CAD build for the part. Positions are in the model's coordinates, mm. A direction names the side the tool comes from. Give positions to 0.01 mm unless a question says otherwise; leave off trailing zeros. Loops run counter-clockwise (first coordinate to the right, second up) from the corner with the lowest first, then second, coordinate; pieces in that order, holes last. Notation, with made-up numbers: M -15.5,82 L -7.5,82 A20 cw -7.5,104 Z; hole C 26.25,-35 d3. An arc over 180 degrees is marked long. One line per question, with ' | ' between items.
```python
from build123d import *

# Parameters (mm, degrees)
F0_R     = 5
F1_DEPTH = 4
F2_DEPTH = 2
F0_R_2   = 2
F3_DEPTH = 16
F4_SIZE  = 0.75
F5_SIZE  = 0.75


with BuildPart() as f1:
    # F0 (on Top) → F1 (new body)
    with BuildSketch(Plane.XY):
        Polygon((-4.5, 20.5), (-4.5, 17.5), (-1.8038475773, 17.5), (-3.375, 18.4071052742), (-3.375, 20.5), align=None)
        Polygon((3.875, 18.4071052742), (2.3038475773, 17.5), (5, 17.5), (5, 20.5), (3.875, 20.5), align=None)
        with BuildLine():
            ThreePointArc((5, 20.5), (0.25, 25.25), (-4.5, 20.5))
            Line((-4.5, 20.5), (-3.375, 20.5))
            Line((-3.375, 20.5), (-3.375, 22.5928947258))
            Line((-3.375, 22.5928947258), (0.25, 24.6857894516))
            Line((0.25, 24.6857894516), (3.875, 22.5928947258))
            Line((3.875, 22.5928947258), (3.875, 20.5))
            Line((3.875, 20.5), (5, 20.5))
        make_face()
        Polygon((-4.5, 17.5), (-17.5, 17.5), (-17.5, -17.5), (-4.5, -17.5), (-2.0538475773, -17.5), (0, -16.3142105484), (2.0538475773, -17.5), (4.5, -17.5), (20.5, -17.5), (20.5, 17.5), (5, 17.5), (2.3038475773, 17.5), (0.25, 16.3142105484), (-1.8038475773, 17.5), align=None)
        Circle(F0_R, mode=Mode.SUBTRACT)
        Polygon((-2.0538475773, -17.5), (-4.5, -17.5), (-4.5, -20.5), (-3.625, -20.5), (-3.625, -18.4071052742), align=None)
        Polygon((4.5, -17.5), (2.0538475773, -17.5), (3.625, -18.4071052742), (3.625, -20.5), (4.5, -20.5), align=None)
        with BuildLine():
            Line((-3.625, -20.5), (-4.5, -20.5))
            ThreePointArc((-4.5, -20.5), (0, -25), (4.5, -20.5))
            Line((4.5, -20.5), (3.625, -20.5))
            Line((3.625, -20.5), (3.625, -22.5928947258))
            Line((3.625, -22.5928947258), (0, -24.6857894516))
            Line((0, -24.6857894516), (-3.625, -22.5928947258))
            Line((-3.625, -22.5928947258), (-3.625, -20.5))
        make_face()
    extrude(amount=F1_DEPTH)

    # F0 (on Top) → F2 (join)
    with BuildSketch(Plane.XY):
        with BuildLine():
            Line((-3.375, 22.5928947258), (-3.375, 20.5))
            Line((-3.375, 20.5), (-1.625, 20.5))
            ThreePointArc((-1.625, 20.5), (0.25, 22.375), (2.125, 20.5))
            Line((2.125, 20.5), (3.875, 20.5))
            Line((3.875, 20.5), (3.875, 22.5928947258))
            Line((3.875, 22.5928947258), (0.25, 24.6857894516))
            Line((0.25, 24.6857894516), (-3.375, 22.5928947258))
        make_face()
        with BuildLine():
            Line((-3.375, 18.4071052742), (-1.8038475773, 17.5))
            Line((-1.8038475773, 17.5), (2.3038475773, 17.5))
            Line((2.3038475773, 17.5), (3.875, 18.4071052742))
            Line((3.875, 18.4071052742), (3.875, 20.5))
            Line((3.875, 20.5), (2.125, 20.5))
            ThreePointArc((2.125, 20.5), (0.25, 18.625), (-1.625, 20.5))
            Line((-1.625, 20.5), (-3.375, 20.5))
            Line((-3.375, 20.5), (-3.375, 18.4071052742))
        make_face()
        Polygon((2.3038475773, 17.5), (-1.8038475773, 17.5), (0.25, 16.3142105484), align=None)
        Polygon((0, -16.3142105484), (-2.0538475773, -17.5), (2.0538475773, -17.5), align=None)
        with BuildLine():
            Line((2.0538475773, -17.5), (-2.0538475773, -17.5))
            Line((-2.0538475773, -17.5), (-3.625, -18.4071052742))
            Line((-3.625, -18.4071052742), (-3.625, -20.5))
            Line((-3.625, -20.5), (-1.875, -20.5))
            ThreePointArc((-1.875, -20.5), (0, -18.625), (1.875, -20.5))
            Line((1.875, -20.5), (3.625, -20.5))
            Line((3.625, -20.5), (3.625, -18.4071052742))
            Line((3.625, -18.4071052742), (2.0538475773, -17.5))
        make_face()
        with BuildLine():
            Line((-1.875, -20.5), (-3.625, -20.5))
            Line((-3.625, -20.5), (-3.625, -22.5928947258))
            Line((-3.625, -22.5928947258), (0, -24.6857894516))
            Line((0, -24.6857894516), (3.625, -22.5928947258))
            Line((3.625, -22.5928947258), (3.625, -20.5))
            Line((3.625, -20.5), (1.875, -20.5))
            ThreePointArc((1.875, -20.5), (0, -22.375), (-1.875, -20.5))
        make_face()
    extrude(amount=F2_DEPTH)

    # F0 (on Top) → F3 (join)
    with BuildSketch(Plane.XY):
        Circle(F0_R)
        Circle(F0_R_2, mode=Mode.SUBTRACT)
    extrude(amount=F3_DEPTH)

    # F4
    f4_edges = [f1.edges().sort_by_distance(p)[0] for p in [
        (-5, 0, 16),
    ]]
    chamfer(f4_edges, length=F4_SIZE)

    # F5
    f5_edges = [f1.edges().sort_by_distance(p)[0] for p in [
        (-1.875, -20.5, 0),
        (-1.625, 20.5, 0),
        (-2, 0, 0),
    ]]
    chamfer(f5_edges, length=F5_SIZE)


solid = f1.part
```
Item 1: Saw through at B-B on z = 5.25. Give the cut face in (x, y), and give its area (3 significant figures).
Conclusion:
outline: C 0,0 d10; hole C 0,0 d4 | area: 66.0 mm²
Item 2: Drill centre lines: line 1 along Y through (x, z) = (0, 10); line 2 along Y through (x, z) = (0.25, 1.65) (3 decimals); line 3 along X through (y, z) = (-20.5, 1.3) (3 decimals). Where is each one in solid material? Low to high. Write a range as [from, to].
Conclusion:
line 1: [-5, -2], [2, 5] | line 2: [-24.993, -22.358], [-18.642, -1.984], [1.984, 18.625], [22.375, 25.25] | line 3: [-4.5, -1.875], [1.875, 4.5]
Item 3: Drop flat-ended pins along their axis: P1, Ø12, axis at x = -13, y = -6.5, coming from the +Z side; P2, Ø0.9, axis at y = -19, z = 2.5, coming from the -X side; P3, Ø3, axis at x = 11, z = 2, coming from the -Y side. Give the stop position or say it passes through.
Conclusion:
P1: z = 4 | P2: x = -4.5 | P3: y = -17.5
Item 4: Saw through at C-C on x = -15. Give the cut face in (y, z).
Conclusion:
outline: M -17.5,0 L 17.5,0 L 17.5,4 L -17.5,4 Z
Item 5: 3-axis set-ups, long thin cutter, end or side, ignore diameter. For faces 5 (the flat face through (5, 19, 2)), 6 (the flat face through (-4.5, -19, 2)), 7 (the flat face through (-3.375, 20, 3)): which of +Z, -Z, +X, -X, +Y, -Y reach the whole face in a straight line?
Conclusion:
face 5: +Z, -Z, +X, +Y | face 6: +Z, -Z, -X, -Y | face 7: +Z
Item 6: Saw through at A-A on y = 0. Give the cut face in (x, z), and give its area (3 significant figures).
Conclusion:
outline: M -17.5,0 L -2.75,0 L -2,0.75 L -2,16 L -4.25,16 L -5,15.25 L -5,4 L -17.5,4 Z; M 2,0.75 L 2.75,0 L 20.5,0 L 20.5,4 L 5,4 L 5,15.25 L 4.25,16 L 2,16 Z | area: 207 mm²
Item 7: Mould opens along X. For faces 1 (the cylindrical face through (-0.41, -18.67, 1.37)), 2 (the flat face through (-11, 17.5, 2)), 3 (the flat face through (4.5, -19, 2)), 4 (the flat face through (-4.5, 19, 2)) say: pulls with the +X half, pulls with the -X half, needs draft (parallel to the pull), parting line crosses it, or undercut.
Conclusion:
face 1: undercut | face 2: needs draft | face 3: pulls with the +X half | face 4: pulls with the -X half
Item 8: Saw through at D-D on y = 13. Give the cut face in (x, z).
Conclusion:
outline: M -17.5,0 L 20.5,0 L 20.5,4 L -17.5,4 Z
